CAD build for the part. Positions are in the model's coordinates, mm. Give positions to 0.01 mm unless a question says otherwise; leave off trailing zeros. Write each loop counter-clockwise with the first axis right and the second up, starting at its lowest first coordinate (ties: lowest second). Pieces come first, ordered by that corner, then holes. Notation, with made-up numbers: (16.5, -6.5) -> (65.5, -6.5) arc R17 cw to (65.5, 8.5) -> close; hole circle Ø7 at (48.5, 49.5). An arc over 180 degrees is marked (long way). Use one line per item in the form item = value. Start each with the question number.
from build123d import *

# Parameters (mm, degrees)
SKETCH2_R           = 2.286
BOSS_EXTRUDE1_DEPTH = 6.35
SKETCH4_R           = 2.286
CUT_EXTRUDE2_DEPTH  = 17.185114529


with BuildPart() as part:
    # Sketch2 → Boss-Extrude1 (new body)
    with BuildSketch(Plane(origin=(0, 0, 0), x_dir=(1, 0, 0), z_dir=(0, 1, 0))):
        with BuildLine():
            Line((0, 4.7625), (14.105106383, 4.7625))
            Line((14.105106383, 4.7625), (14.105106383, -4.7625))
            Line((14.105106383, -4.7625), (0, -4.7625))
            ThreePointArc((0, -4.7625), (-4.7625, 0), (0, 4.7625))
        make_face()
        with Locations(Location((0, 0, 0), (0, 0, 270))):
            Circle(SKETCH2_R, mode=Mode.SUBTRACT)
    extrude(amount=BOSS_EXTRUDE1_DEPTH)

    # Sketch4 → Cut-Extrude2 (cut, through all)
    with BuildSketch(Plane(origin=(0, 6.35, 0), x_dir=(1, 0, 0), z_dir=(0, 1, 0))):
        with BuildLine():
            Line((14.105106383, 4.7625), (9.342606383, 4.7625))
            ThreePointArc((9.342606383, 4.7625), (12.710202422, 3.367596052), (14.105106383, 1.8e-08))
            Line((14.105106383, 1.8e-08), (14.105106383, 4.7625))
        make_face()
        with BuildLine():
            Line((14.105106383, -4.7625), (14.105106383, 1.8e-08))
            ThreePointArc((14.105106383, 1.8e-08), (12.710202435, -3.367596039), (9.342606383, -4.7625))
            Line((9.342606383, -4.7625), (14.105106383, -4.7625))
        make_face()
        with Locations(Location((9.342606383, 0, 0), (0, 0, 270))):
            Circle(SKETCH4_R)
    extrude(amount=-CUT_EXTRUDE2_DEPTH, mode=Mode.SUBTRACT)


solid = part.part
1) Cut at D-D (z = 2). Give the cut face in (x, y).
2) Two-plate mould, pull along X, no slides. Class faces 1 (the face through (-2.03, 3.13, 1.05)), 2 (the face through (5, 6.35, 0)), 3 (the face through (-4.76, 3.13, 0.1)): released by +X, released by -X, zero draft, split by the parting line, or undercut.
3) Cut at C-C (z = -1). Give the cut face in (x, y).
4) Cut at A-A (y = 3.75). Give the cut face in (x, z) (1 decimal), and give its area (3 significant figures).
5) Wall check: line 1 along X through (y, z) = (3.5, 0); line 2 along X through (y, z) = (2, 1.75); line 3 along Z through (x, y) = (8, 5.5). Give the ranges that are in metal, low to high. Write a range as from..to.
6) Pin check, flat tip, straight feed: pin 1 (1.5 mm diameter, centred on y = 3.5, z = -3, fed in from +X). Stop position of the tip, or through.
7) Cut at B-B (x = -1.25). Give the cut face in (y, z), and give its area (3 significant figures).
Final values:
q1.outline = (-4.32, 0) -> (-1.11, 0) -> (-1.11, 6.35) -> (-4.32, 6.35) -> close; (1.11, 0) -> (8.24, 0) -> (8.24, 6.35) -> (1.11, 6.35) -> close; (10.45, 0) -> (13.66, 0) -> (13.66, 6.35) -> (10.45, 6.35) -> close
q2.face_1 = undercut
q2.face_2 = zero draft
q2.face_3 = released by -X
q3.outline = (-4.66, 0) -> (-2.06, 0) -> (-2.06, 6.35) -> (-4.66, 6.35) -> close; (2.06, 0) -> (7.29, 0) -> (7.29, 6.35) -> (2.06, 6.35) -> close; (11.4, 0) -> (14, 0) -> (14, 6.35) -> (11.4, 6.35) -> close
q4.outline = (0, -4.8) -> (9.3, -4.8) arc R4.8 ccw to (9.3, 4.8) -> (0, 4.8) arc R4.8 ccw to start; hole circle Ø4.6 at (0, 0); hole circle Ø4.6 at (9.3, 0)
q4.area = 127 mm^2
q5.line_1 = -4.76..-2.29, 2.29..7.06, 11.63..14.11
q5.line_2 = -4.43..-1.47, 1.47..7.87, 10.81..13.77
q5.line_3 = -4.76..-1.85, 1.85..4.76
q6.pin_1 = 13.54
q7.outline = (0, -4.6) -> (6.35, -4.6) -> (6.35, -1.91) -> (0, -1.91) -> close; (0, 1.91) -> (6.35, 1.91) -> (6.35, 4.6) -> (0, 4.6) -> close
q7.area = 34.1 mm^2
